Geometry check sheet. Reference: the model listing, model coordinates, mm. Face numbers are marked on the shaded views. A direction names the side the tool comes from. Round coordinates to 2 decimals unless told otherwise and drop trailing zeros. Write each loop counter-clockwise with the first axis right and the second up, starting at its lowest first coordinate (ties: lowest second). Pieces come first, ordered by that corner, then holes. Notation, with made-up numbers: M -8,70 L 45,70 A19 cw 45,105 Z; hole C 39.25,-34.75 d6. An arc over 180 degrees is marked long. One line per item, written item: value. Start each with the question number.
1. Section check B-B (x = 0). Record the boundary of the cut face in (y, z), and give its area (3 significant figures).
2. Scan lines: probe 1 along X at (y, z) = (-5.25, 9); probe 2 along Y at (x, z) = (12.5, 26); probe 3 along X at (y, z) = (8.25, 53.5). Record each from-to range of solid material in increasing order. Write a range as [from, to].
3. Section check A-A (y = -7.5). Record the boundary of the cut face in (x, z), and give its area (3 significant figures).
4. Section check C-C (z = 52). Record the boundary of the cut face in (x, y).
5. Depth check by flat-ended pin: P1, Ø4.5, axis at x = 13, y = -7, coming from the +Z side; P2, Ø1, axis at x = 11.5, z = 45, coming from the -Y side; P3, Ø8, axis at y = 0.5, z = 31.5, coming from the -X side. Enter the tip coordinate at first touch or a pass-through.
6. Section check D-D (x = 14.5). Record the boundary of the cut face in (y, z), and give its area (3 significant figures).
7. Access from +Z, -Z, +X, -X, +Y, -Y to the whole of each face (thin tool, end or side, straight path). Record for the marked faces 1, 2 and 3.
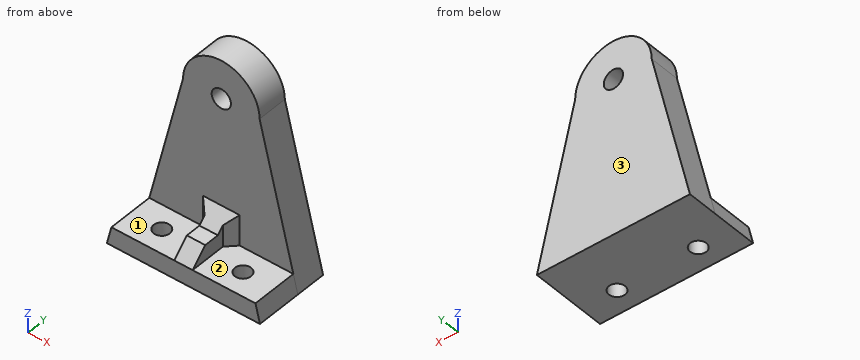
Solid Edge part; units mm, degrees
sketch "Sketch1" plane through (0, 0, 0) normal (0, -1, 0) x (1, 0, 0)
  circle A0 centre (0, 51) radius 3.15
  line L0 (25, 0) -> (12.5, 51)
  line L1 (0, 0) -> (25, 0)
  line L2 (0, 0) -> (-25, 0)
  line L3 (-25, 0) -> (-12.5, 50.9918)
  arc A1 (-12.5, 50.9918) -> (12.5, 51) centre (0, 51) cw
extrude "Protrusion1" add sketch "Sketch1" against normal blind 10
sketch "Sketch2" plane through (0, 0, 31.75) normal (0, -1, 0) x (1, 0, 0)
  line L0 (0, -25.75) -> (23.5294, -25.75)
  line L1 (23.5294, -25.75) -> (25, -31.75)
  line L2 (25, -31.75) -> (-25, -31.75)
  line L3 (-25, -31.75) -> (-23.5292, -25.75)
  line L4 (-23.5292, -25.75) -> (0, -25.75)
extrude "ExtrudedProtrusion_3" add sketch "Sketch2" along normal blind 15
sketch "Sketch3" plane through (0.0001, -7.5, 6) normal (0, 0, 1) x (1, 0, 0)
  line L0 (2.9999, -7.5) -> (2.9999, 7.5)
  line L1 (2.9999, 7.5) -> (-3.0001, 7.5)
  line L2 (-3.0001, 7.5) -> (-3.0001, -7.5)
  line L3 (-3.0001, -7.5) -> (2.9999, -7.5)
extrude "ExtrudedProtrusion_4" add sketch "Sketch3" along normal blind 5
chamfer "Chamfer_1" distance 5 angle 45 2 edges at (0, 0, 11) (0, -15, 11)
chamfer "Chamfer_2" distance 3 angle 45 2 edges at (3, 0, 11) (-3, 0, 11)
sketch "Sketch4" plane through (-13.2646, -7.5, 6) normal (0, 0, 1) x (1, 0, 0)
  circle A0 centre (26.5293, 0) radius 2.65
  circle A1 centre (0, 0) radius 2.65
extrude "Cutout1" cut sketch "Sketch4" against normal up to next
Result sheet:
1. outline: M -15,0 L 10,0 L 10,47.85 L 0,47.85 L 0,16 L -5,11 L -10,11 L -15,6 Z; M 0,54.15 L 10,54.15 L 10,63.5 L 0,63.5 Z
1. area: 737 mm2
2. probe 1: x = [-3, 3]
2. probe 2: y = [0, 10]
2. probe 3: x = [-12.25, -1.92], [1.92, 12.25]
3. outline: M -25,0 L -15.91,0 L -15.91,6 L -23.53,6 Z; M -10.61,0 L 10.61,0 L 10.61,6 L 3,6 L 3,11 L -3,11 L -3,6 L -10.61,6 Z; M 15.91,0 L 25,0 L 23.53,6 L 15.91,6 Z
3. area: 258 mm2
4. outline: M -12.46,0 L -2.99,0 L -2.99,10 L -12.46,10 Z; M 2.99,0 L 12.46,0 L 12.46,10 L 2.99,10 Z
5. P1: stops at z = 6
5. P2: stops at y = 0
5. P3: stops at x = -18.26
6. outline: M -15,0 L -9.84,0 L -9.84,6 L -15,6 Z; M -5.16,0 L 10,0 L 10,42.84 L 0,42.84 L 0,6 L -5.16,6 Z
6. area: 490 mm2
7. face 1: +Z, -X, -Y
7. face 2: +Z, +X, -Y
7. face 3: +Z, -Z, +X, -X, +Y
